Could you check a few things on this model? Use its own coordinates, in mm. Round coordinates to 2 decimals unless told otherwise and drop trailing zeros. Loops run counter-clockwise (first coordinate to the right, second up) from the corner with the lowest first, then second, coordinate; pieces in that order, holes last. Notation, with made-up numbers: (8.25, 53.25) -> (48.25, 53.25) arc R23 ccw to (48.25, 65.25) -> close; hole circle Ø3 at (22.25, 57.5). An arc over 180 degrees is marked (long way). One line per item, written item: value.
```python
from build123d import *

# Parameters (mm, degrees)
F0_R     = 3.175
F1_DEPTH = 3.175


with BuildPart() as f1:
    # F0 (on Right) → F1 (new body)
    with BuildSketch(Plane.YZ):
        with BuildLine():
            Line((-0.683293, -22.206229), (-21.279692, -6.062372))
            ThreePointArc((-21.279692, -6.062372), (-31.89988, -6.809987), (-32.223099, -17.45155))
            Line((-32.223099, -17.45155), (-32.127586, -17.5618))
            Line((-32.127586, -17.5618), (-3.144408, -51.016742))
            ThreePointArc((-3.144408, -51.016742), (4.260096, -54.808331), (12.221904, -52.397431))
            Line((12.221904, -52.397431), (59.870195, -14.049133))
            Line((59.870195, -14.049133), (63.249417, -11.329467))
            ThreePointArc((63.249417, -11.329467), (62.611086, 11.0927), (40.187851, 10.493082))
            ThreePointArc((40.187851, 10.493082), (40.178419, 10.48314), (40.168995, 10.47319))
            Line((40.168995, 10.47319), (10.036033, -21.370629))
            ThreePointArc((10.036033, -21.370629), (4.839042, -23.875239), (-0.683293, -22.206229))
        make_face()
        with Locations((5.254567, -43.740418)):
            Circle(F0_R, mode=Mode.SUBTRACT)
        with Locations((-26.176328, -12.30952)):
            Circle(F0_R, mode=Mode.SUBTRACT)
        with Locations((51.699796, -0.4381)):
            Circle(F0_R, mode=Mode.SUBTRACT)
    extrude(amount=F1_DEPTH)


solid = f1.part
```
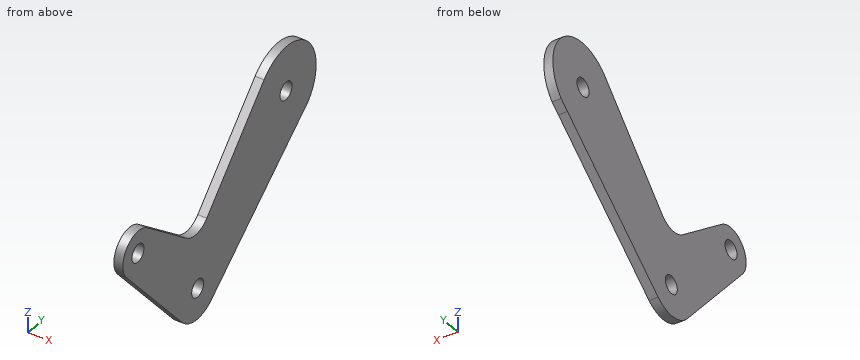
(1) Imagine slicing it at B-B on y = 4.5. Write out the boundary of the cut face in (x, z) (3 decimals).
Results below:
outline: (0, -54.827) -> (3.175, -54.827) -> (3.175, -46.824) -> (0, -46.824) -> close; (0, -40.656) -> (3.175, -40.656) -> (3.175, -23.894) -> (0, -23.894) -> close
(2) For pin 1 Ø1.5 at (x, y) = (1.5, -1.5) entering from -Z, with a flat end and sliding along its axis, tell me the tip position at first contact or that it passes through.
Results below:
pin 1: stops at z = -53.09
(3) Imagine slicing it at C-C on y = 38. Write out the boundary of the cut face in (x, z) (3 decimals).
Results below:
outline: (0, -31.651) -> (3.175, -31.651) -> (3.175, 8.181) -> (0, 8.181) -> close
(4) Imagine slicing it at D-D on z = -27. Write out the boundary of the cut face in (x, y) (3 decimals), then the cut area to 3 significant figures.
Results below:
outline: (0, -23.951) -> (3.175, -23.951) -> (3.175, 43.779) -> (0, 43.779) -> close
area: 215 mm²
(5) Imagine slicing it at A-A on x = 2.6. Give the number of separate pieces and of enclosed holes in the cut face, then the cut area to 3 significant figures.
Results below:
separate pieces: 1
enclosed holes: 3
area: 2,990 mm²
(6) Please list where these lines run through material, in increasing order: L1, parallel to Y at x = 0.75, z = -11; L2, parallel to Y at x = 2.85, z = -3; L3, parallel to Y at x = 2.05, z = -2.
Results below:
L1: y = -34.01 to -29.07, -23.28 to -14.98, 19.85 to 63.55
L2: y = 27.42 to 49.82, 53.58 to 67.37
L3: y = 28.37 to 48.94, 54.46 to 67.5
